from build123d import *

# Parameters (mm, degrees)
F1_DEPTH = 5


with BuildPart() as f1:
    # F0 (on Front) → F1 (new body)
    with BuildSketch(Plane.XZ):
        with BuildLine():
            ThreePointArc((22.2689937055, 5.6673698127), (9.8946250347, 10.793001142), (4.7689937055, 23.1673698127))
            Line((4.7689937055, 23.1673698127), (-57.7310062945, 23.1673698127))
            ThreePointArc((-57.7310062945, 23.1673698127), (-52.4699634864, 21.6715704554), (-48.7828135685, 17.631655527))
            ThreePointArc((-48.7828135685, 17.631655527), (-4.6979977055, -3.7996215983), (16.7332794198, -47.8844374613))
            ThreePointArc((16.7332794198, -47.8844374613), (20.7731943482, -51.5715873792), (22.2689937055, -56.8326301873))
            Line((22.2689937055, -56.8326301873), (22.2689937055, 5.6673698127))
        make_face()
        with BuildLine():
            ThreePointArc((-49.4029892828, 7.631655527), (-53.0064503819, 4.3538250418), (-57.7310062945, 3.1673698127))
            ThreePointArc((-57.7310062945, 3.1673698127), (-15.3045994233, -14.4062233161), (2.2689937055, -56.8326301873))
            ThreePointArc((2.2689937055, -56.8326301873), (3.4554489346, -52.1080742747), (6.7332794198, -48.5046131756))
            ThreePointArc((6.7332794198, -48.5046131756), (-11.7690655174, -10.8706894101), (-49.4029892828, 7.631655527))
        make_face()
        with BuildLine():
            ThreePointArc((6.7332794198, -48.5046131756), (3.4554489346, -52.1080742747), (2.2689937055, -56.8326301873))
            Line((2.2689937055, -56.8326301873), (7.2689937055, -56.8326301873))
            ThreePointArc((7.2689937055, -56.8326301873), (7.1349268732, -52.6600153853), (6.7332794198, -48.5046131756))
        make_face()
        with BuildLine():
            ThreePointArc((2.2689937055, -56.8326301873), (12.2689937055, -66.8326301873), (22.2689937055, -56.8326301873))
            Line((22.2689937055, -56.8326301873), (17.2689937055, -56.8326301873))
            ThreePointArc((17.2689937055, -56.8326301873), (12.2689937055, -61.8326301873), (7.2689937055, -56.8326301873))
            Line((7.2689937055, -56.8326301873), (2.2689937055, -56.8326301873))
        make_face()
        with BuildLine():
            Line((17.2689937055, -56.8326301873), (22.2689937055, -56.8326301873))
            ThreePointArc((22.2689937055, -56.8326301873), (20.7731943482, -51.5715873792), (16.7332794198, -47.8844374613))
            ThreePointArc((16.7332794198, -47.8844374613), (17.134945341, -52.3505229023), (17.2689937055, -56.8326301873))
        make_face()
        with BuildLine():
            Line((-57.7310062945, 18.1673698127), (-57.7310062945, 23.1673698127))
            ThreePointArc((-57.7310062945, 23.1673698127), (-67.7310062945, 13.1673698127), (-57.7310062945, 3.1673698127))
            Line((-57.7310062945, 3.1673698127), (-57.7310062945, 8.1673698127))
            ThreePointArc((-57.7310062945, 8.1673698127), (-62.7310062945, 13.1673698127), (-57.7310062945, 18.1673698127))
        make_face()
        with BuildLine():
            ThreePointArc((-48.7828135685, 17.631655527), (-52.4699634864, 21.6715704554), (-57.7310062945, 23.1673698127))
            Line((-57.7310062945, 23.1673698127), (-57.7310062945, 18.1673698127))
            ThreePointArc((-57.7310062945, 18.1673698127), (-53.2488990095, 18.0333214482), (-48.7828135685, 17.631655527))
        make_face()
        with BuildLine():
            Line((-57.7310062945, 8.1673698127), (-57.7310062945, 3.1673698127))
            ThreePointArc((-57.7310062945, 3.1673698127), (-53.0064503819, 4.3538250418), (-49.4029892828, 7.631655527))
            ThreePointArc((-49.4029892828, 7.631655527), (-53.5583914925, 8.0333029804), (-57.7310062945, 8.1673698127))
        make_face()
        with BuildLine():
            Line((12.2689937055, 23.1673698127), (4.7689937055, 23.1673698127))
            ThreePointArc((4.7689937055, 23.1673698127), (9.8946250347, 10.793001142), (22.2689937055, 5.6673698127))
            Line((22.2689937055, 5.6673698127), (22.2689937055, 13.1673698127))
            ThreePointArc((22.2689937055, 13.1673698127), (15.1979258936, 16.0963020009), (12.2689937055, 23.1673698127))
        make_face()
        with BuildLine():
            ThreePointArc((22.2689937055, 5.6673698127), (34.6433623763, 10.793001142), (39.7689937055, 23.1673698127))
            ThreePointArc((39.7689937055, 23.1673698127), (22.2689937055, 40.6673698127), (4.7689937055, 23.1673698127))
            Line((4.7689937055, 23.1673698127), (12.2689937055, 23.1673698127))
            ThreePointArc((12.2689937055, 23.1673698127), (22.2689937055, 33.1673698127), (32.2689937055, 23.1673698127))
            ThreePointArc((32.2689937055, 23.1673698127), (29.3400615174, 16.0963020009), (22.2689937055, 13.1673698127))
            Line((22.2689937055, 13.1673698127), (22.2689937055, 5.6673698127))
        make_face()
    extrude(amount=F1_DEPTH)


solid = f1.part
Build history of the part. All positions in model axes, mm. A direction names the side the tool comes from. Round coordinates to 2 decimals unless told otherwise and drop trailing zeros. Loops run counter-clockwise (first coordinate to the right, second up) from the corner with the lowest first, then second, coordinate; pieces in that order, holes last. Notation, with made-up numbers: (-10.5, 85) -> (-6.5, 85) arc R23 cw to (-6.5, 124) -> close; hole circle Ø3 at (46, 19.5). An arc over 180 degrees is marked (long way). Answer in a Markdown table with one row per item.
Item 1: Saw through at C-C (z = -50). Write the cut outline in (x, y), and give its area (3 significant figures).
Answers below:
| item | result |
|---|---|
| outline | (1.88, -5) -> (6.91, -5) -> (6.91, 0) -> (1.88, 0) -> close; (16.96, -5) -> (22.27, -5) -> (22.27, 0) -> (16.96, 0) -> close |
| area | 51.7 mm² |
Item 2: Mould opens along Z. For faces 1 (the cylindrical face through (12.38, -2.46, -61.83)), 2 (the cylindrical face through (-62.73, -2.46, 13.06)), 3 (the cylindrical face through (-67.73, -2.46, 13.39)), 4 (the flat face through (2, -5, -1)) say: +Z half, -Z half, draft (parallel to the pull), parting line (faces both ways), or undercut.
Answers below:
| item | result |
|---|---|
| face 1 | undercut |
| face 2 | undercut |
| face 3 | parting line |
| face 4 | draft |
Item 3: Pin check, flat tips, straight feed: pin 1 (3 mm diameter, centred on x = -42.5, y = -1, fed in from -Z); pin 2 (2.5 mm diameter, centred on y = -2.5, z = -36, fed in from +X); pin 3 (2 mm diameter, centred on x = -35.5, z = 26, fed in from -Y); pin 4 (1.5 mm diameter, centred on x = -56, y = -3.5, fed in from -Z). Stop position of each tip, or through.
Answers below:
| item | result |
|---|---|
| pin 1 | stops at z = 0.79 |
| pin 2 | stops at x = 22.27 |
| pin 3 | passes through |
| pin 4 | stops at z = 3.12 |
Item 4: Drill centre lines: L1, parallel to X at y = -4.65, z = -38; L2, parallel to X at y = -2.2, z = 28; L3, parallel to Z at x = -6, y = -2.5. Where is each one in solid material? Low to high. Write a range as [from, to].
Answers below:
| item | result |
|---|---|
| L1 | x = [-0.76, 4.48], [14.87, 22.27] |
| L2 | x = [5.45, 13.51], [31.02, 39.09] |
| L3 | z = [-26.44, -17.48], [-2.53, 23.17] |
Item 5: Saw through at A-A (y = -3.9). Write the cut outline in (x, z), and give its area (3 significant figures).
Answers below:
| item | result |
|---|---|
| outline | (-57.73, 3.17) arc R60 cw to (2.27, -56.83) arc R10 ccw to (22.27, -56.83) -> (22.27, 5.67) arc R17.5 ccw (long way) to (4.77, 23.17) -> (-57.73, 23.17) arc R10 ccw to start; hole (-57.73, 8.17) arc R65 cw to (7.27, -56.83) arc R5 ccw to (17.27, -56.83) arc R75 ccw to (-57.73, 18.17) arc R5 ccw to start; hole circle Ø20 at (22.27, 23.17) |
| area | 3,120 mm² |
Item 6: Saw through at B-B (x = -56.5). Write the cut outline in (y, z).
Answers below:
| item | result |
|---|---|
| outline | (-5, 3.15) -> (0, 3.15) -> (0, 8.16) -> (-5, 8.16) -> close; (-5, 18.16) -> (0, 18.16) -> (0, 23.17) -> (-5, 23.17) -> close |
Item 7: Which spindle directions (+Z, -Z, +X, -X, +Y, -Y) get a long thin tool onto all of the face, cutting with end or side? Do faces 5 (the cylindrical face through (-15.774, -2.465, -13.942)), 6 (the flat face through (-26, -2, 23.167)), 7 (the flat face through (22.269, -2, -26)). Say none if no direction does.
Answers below:
| item | result |
|---|---|
| face 5 | -Z, -X, +Y, -Y |
| face 6 | +Z, -X, +Y, -Y |
| face 7 | -Z, +X, +Y, -Y |
